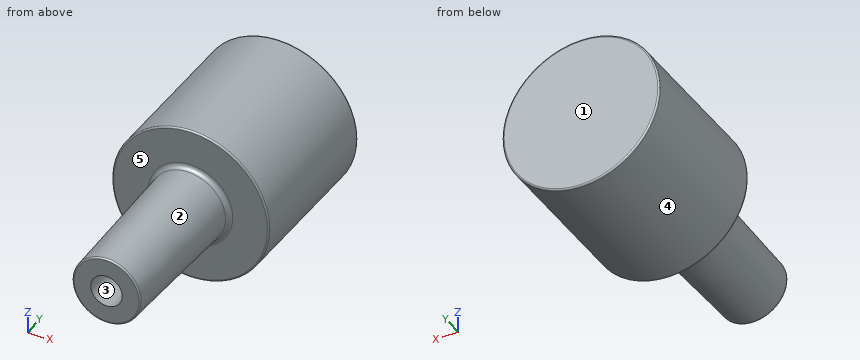
```python
from build123d import *

# Parameters (mm, degrees)
F3_D     = 5.1054
F3_DEPTH = 22.225
F3_TIP   = 1.5338169022
F4_R     = 0.762
F5_R     = 0.254


with BuildPart() as f1:
    # F0 (on Right) → F1 (revolve)
    with BuildSketch(Plane.YZ):
        Polygon((-24.13, 0), (25.4, 0), (25.4, 12.7), (0, 12.7), (0, 6.096), (-24.13, 5.4941811878), align=None)
    revolve(axis=Axis((0, 0.635, 0), (0, 1, 0)))

    # F3
    with Locations(Plane.XZ.offset(24.13)):
        with Locations((0, 0)):
            Hole(F3_D / 2, depth=F3_DEPTH)
            with Locations((0, 0, -(F3_DEPTH + F3_TIP / 2))):  # 118° drill point
                Cone(0, F3_D / 2, F3_TIP, mode=Mode.SUBTRACT)

    # F4
    f4_edges = [f1.edges().sort_by_distance(p)[0] for p in [
        (0, 0, -6.096),
    ]]
    fillet(f4_edges, radius=F4_R)

    # F5
    f5_edges = [f1.edges().sort_by_distance(p)[0] for p in [
        (0, 0, -12.7),
        (0, 25.4, -12.7),
        (0, -24.13, -5.494181),
    ]]
    fillet(f5_edges, radius=F5_R)


solid = f1.part
```
Geometry: final body of the model. Coordinates: model frame, mm. Face numbers are marked on the shaded views. A direction names the side the tool comes from. Coordinates: 2 decimals unless noted, no trailing zeros. Order: outer loops, then holes, each group sorted by start corner. A loop starts at its lowest first (then second) coordinate and runs counter-clockwise, first axis right, second up. Notation, with made-up numbers: (-1, 32.25) - (24, 32.25) arc R18 ccw to (24, 58.25) - close; hole circle Ø4 at (75, 34). An arc over 180 degrees is marked (long way). Write each question's results on one line, items separated by ' | '.
(1) Set-up query: the marked faces 1 and 2. Return all of +Z, -Z, +X, -X, +Y, -Y with unobstructed straight access to the full face (end or side cutting, diameter ignored); none if empty.
Values found:
face 1: +Z, -Z, +X, -X, +Y | face 2: -Y
(2) Mould query, pull axis X, two halves, no side actions, for the marked faces 3, 4 and 5. Classes: +X half, -X half, draft (parallel to the pull), parting line (faces both ways), or undercut.
Values found:
face 3: undercut | face 4: parting line | face 5: draft
(3) First-contact query: pin 1 Ø6 at (y, z) = (-17.5, -3) entering from +X; pin 2 Ø2 at (x, y) = (8, 1.5) entering from -Z; pin 3 Ø3 at (x, y) = (3.5, -8) entering from -Z. Flat tips, straight axial feed; report the tip coordinate or a pass-through.
Values found:
pin 1: stops at x = 5.68 | pin 2: stops at z = -10.6 | pin 3: stops at z = -5.55
(4) Section query B-B, the plane y = 16. Return the cut outline in (x, z), plus the area to 3 significant figures.
Values found:
outline: circle Ø25.4 at (0, 0) | area: 507 mm²
(5) Section query A-A, the plane y = -11. Return the cut outline in (x, z), plus the area to 3 significant figures.
Values found:
outline: circle Ø11.64 at (0, 0); hole circle Ø5.11 at (0, 0) | area: 86.0 mm²
(6) Line query: line 1 (Y direction, x = 4.25, z = -10.75); line 2 (Z direction, x = 0, y = -15.5); line 3 (Z direction, x = 0, y = -18.75). Output: solid intervals per line, ascending. Write a range as [from, to].
Values found:
line 1: y = [0, 25.4] | line 2: z = [-5.71, -2.55], [2.55, 5.71] | line 3: z = [-5.63, -2.55], [2.55, 5.63]
